Source: CAD feature listing. Evaluate the final solid. Frame: model axes, mm. Coordinates: 2 decimals unless noted, no trailing zeros. Order: outer loops, then holes, each group sorted by start corner. A loop starts at its lowest first (then second) coordinate and runs counter-clockwise, first axis right, second up.
Autodesk Fusion 360 part; units mm, degrees
sketch "Sketch1" plane through (0, 0, 0) normal (0, 0, 1) x (1, 0, 0)
  line L0 (0, 0) -> (300, 0)
  line L1 (300, 0) -> (300, 335)
  line L2 (300, 335) -> (0, 335)
  line L3 (0, 335) -> (0, 0)
  line L4 (0, 0) -> (100, 0)
  line L5 (100, 0) -> (100, 60)
  line L6 (100, 60) -> (0, 60)
  line L7 (0, 60) -> (0, 0)
  line L8 (300, 0) -> (280, 0)
  line L9 (280, 0) -> (280, 60)
  line L10 (280, 60) -> (300, 60)
  line L11 (300, 60) -> (300, 0)
  line L12 (0, 335) -> (300, 335)
  line L13 (300, 335) -> (300, 670)
  line L14 (300, 670) -> (0, 670)
  line L15 (0, 670) -> (0, 335)
  line L16 (0, 670) -> (20, 670)
  line L17 (20, 670) -> (20, 570)
  line L18 (20, 570) -> (0, 570)
  line L19 (0, 570) -> (0, 670)
  circle A0 centre (20, 570) radius 4.5
  circle A1 centre (280, 60) radius 4.5
  circle A2 centre (100, 60) radius 4.5
  line L20 (20, 570) -> (20, 530)
  line L21 (20, 530) -> (74, 530)
  line L22 (74, 530) -> (74, 410)
  line L23 (74, 410) -> (20, 410)
  line L24 (20, 410) -> (20, 530)
  line L25 (0, 335) -> (124, 335)
  line L26 (124, 335) -> (124, 121.3118)
  line L27 (124, 121.3118) -> (0, 121.3118)
  line L28 (0, 121.3118) -> (0, 335)
  circle A3 centre (124, 121.3118) radius 0.5
  line L29 (124, 121.3118) -> (164, 121.3118)
  line L30 (164, 121.3118) -> (164, 81.3118)
  line L31 (164, 81.3118) -> (124, 81.3118)
  line L32 (124, 81.3118) -> (124, 121.3118)
  circle A4 centre (164, 121.3118) radius 0.5
  circle A5 centre (164, 81.3118) radius 0.5
  circle A6 centre (124, 81.3118) radius 0.5
  line L33 (47, 530) -> (47, 537.5)
  circle A7 centre (47, 537.5) radius 0.5
  line L34 (47, 410) -> (47, 402.5)
  circle A8 centre (47, 402.5) radius 0.5
  line L35 (0, 335) -> (295.006, 335)
  line L36 (295.006, 335) -> (295.006, -131.766)
  line L37 (295.006, -131.766) -> (0, -131.766)
  line L38 (0, -131.766) -> (0, 335)
  line L39 (-10, 345) -> (305.006, 345)
  line L40 (305.006, 340.5643) -> (305.006, -131.766)
  line L41 (295.006, -141.766) -> (0, -141.766)
  line L42 (-10, -131.766) -> (-10, 345)
  circle A9 centre (20, 570) radius 24.5
  circle A10 centre (100, 60) radius 24.5
  circle A11 centre (280, 60) radius 24.5
  line L43 (301.7178, 347.9772) -> (36.444, 588.1617)
  line L44 (-10, 345) -> (-4.4927, 570.5979)
  arc A12 (-10, -131.766) -> (0, -141.766) centre (0, -131.766) ccw
  arc A13 (295.006, -141.766) -> (305.006, -131.766) centre (295.006, -131.766) ccw
  arc A14 (305.006, 340.5643) -> (301.7178, 347.9772) centre (295.006, 340.5643) ccw
  dimension "d1" = 300
  dimension "d2" = 335
  dimension "d3" = 100
  dimension "d4" = 60
  dimension "d5" = 20
  dimension "d6" = 60
  dimension "d7" = 300
  dimension "d8" = 335
  dimension "d9" = 20
  dimension "d10" = 100
  dimension "d11" = 9
  dimension "d12" = 9
  dimension "d13" = 9
  dimension "d14" = 40
  dimension "d15" = 54
  dimension "d16" = 120
  dimension "d17" = 124
  dimension "d18" = 213.6882
  dimension "d19" = 1
  dimension "d20" = 40
  dimension "d21" = 40
  dimension "d22" = 1
  dimension "d23" = 1
  dimension "d24" = 1
  dimension "d25" = 7.5
  dimension "d26" = 1
  dimension "d27" = 7.5
  dimension "d28" = 1
  dimension "d29" = 295.006
  dimension "d30" = 466.766
  dimension "d32" = 20
  dimension "d33" = 20
  dimension "d34" = 20
  dimension "d35" = 10
  dimension "d36" = 10
extrude "Extrude1" add sketch "Sketch1" along normal blind 6 contours L0 L3 L4 L5 L6 L7 L38 A10 | L0 L1 L3 L7 L8 L11 L13 L15 L28 L36 L37 L38 L39 L40 L41 L42 A11 A12 A13 A14 | L0 L4 L8 L36 L37 L38 | L0 L2 L3 L5 L6 L9 L12 L26 L27 A3 L29 L30 L31 L32 A4 A5 A6 L35 L36 L38 A10 A11 | L0 L8 L9 L36 A11 | L5 L6 A2 A10 | L5 L6 A2 A10 | L2 L3 L12 L25 L26 L27 L28 A3 L35 L38 | L0 L1 L8 L11 L36 A11 | L9 L10 A1 L36 A11 | L9 L10 A1 L36 A11 | L2 L12 L13 L15 L25 L35 L39 | L1 L10 L11 L36 A11 | L1 L10 L36 A11 | L1 L2 L12 L36 A11 | L15 L39 A9 L44 | L21 L22 L23 L24 | L13 L15 L39 A9 L43 | A3 L29 L30 L31 L32 A4 A5 A6 | L1 L11 A11 | L15 L19 A9 | L15 L18 A0 L20 A9 | L13 L39 L43 A14 | L15 L17 L18 L19 A0 A9 | L17 A0 L20 A9
sketch "FaceSketch" plane through (0, 0, 6) normal (0, 0, 1) x (-1, 0, 0)
  circle A0 centre (-124, -81.3118) radius 0.5
  circle A1 centre (-164, -121.3118) radius 0.5
  circle A2 centre (-280, -60) radius 4.5
  circle A3 centre (-20, -570) radius 4.5
  circle A4 centre (-47, -402.5) radius 0.5
  circle A5 centre (-124, -121.3118) radius 0.5
  circle A6 centre (-47, -537.5) radius 0.5
  circle A7 centre (-100, -60) radius 4.5
  circle A8 centre (-164, -81.3118) radius 0.5
  arc A9 (-295.006, 141.766) -> (-305.006, 131.766) centre (-295.006, 131.766) ccw
  line L0 (-305.006, 131.766) -> (-305.006, -340.5643)
  arc A10 (-305.006, -340.5643) -> (-301.7178, -347.9772) centre (-295.006, -340.5643) ccw
  line L1 (-301.7178, -347.9772) -> (-36.444, -588.1617)
  arc A11 (-36.444, -588.1617) -> (4.4927, -570.5979) centre (-20, -570) ccw
  line L2 (4.4927, -570.5979) -> (10, -345)
  line L3 (10, -345) -> (10, 131.766)
  arc A12 (10, 131.766) -> (0, 141.766) centre (0, 131.766) ccw
  line L4 (0, 141.766) -> (-295.006, 141.766)
equation "d19 = d26"
equation "d22 = d19"
equation "d23 = d19"
equation "d24 = d19"
equation "d28 = d26"
1. Pin query (flat end, axial travel): P1, Ø8, axis at x = 280, y = 60, coming from the -Z side; P2, Ø1.5, axis at x = 132.5, z = 4, coming from the +Y side; P3, Ø1, axis at y = 461.5, z = 1.5, coming from the +X side. Return the tip coordinate at first contact, or that it passes through.
Findings:
P1: passes through
P2: stops at y = 501.87
P3: stops at x = 176.89
2. Section query C-C on x = 267. Return loops of the section in (y, z), plus the area to 3 significant figures.
Findings:
outline: (-141.77, 0) - (379.41, 0) - (379.41, 6) - (-141.77, 6) - close
area: 3,130 mm2
3. Section query B-B on x = 227. Return loops of the section in (y, z).
Findings:
outline: (-141.77, 0) - (415.63, 0) - (415.63, 6) - (-141.77, 6) - close
4. Ray query, line 1 (X direction, y = 570, z = 4); line 2 (Y direction, x = 22, z = 2.8); line 3 (Y direction, x = 100, z = 1.95). Return the intervals inside material, ascending.
Findings:
line 1: x = -4.51 to 15.5, 24.5 to 56.5
line 2: y = -141.77 to 565.97, 574.03 to 594.42
line 3: y = -141.77 to 55.5, 64.5 to 530.62
5. Section query A-A on z = 1.75. Count the separate pieces of the cut face and the enclosed holes in it, plus the area to 3 significant figures.
Findings:
separate pieces: 1
enclosed holes: 9
area: 196,000 mm2
